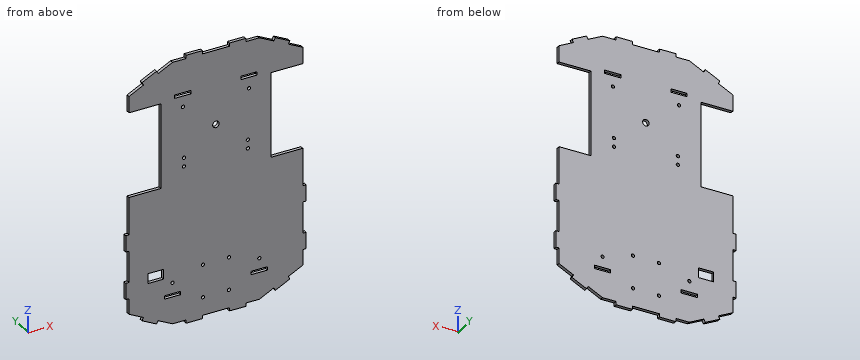
from build123d import *

# Parameters (mm, degrees)
SKETCH1_R           = 1.5
SKETCH1_R_2         = 3
SKETCH1_W           = 15.1
SKETCH1_H           = 3.1
SKETCH1_W_2         = 14
SKETCH1_H_2         = 9
BOSS_EXTRUDE1_DEPTH = 3


with BuildPart() as part:
    # Sketch1 → Boss-Extrude1 (new body)
    with BuildSketch(Plane(origin=(0, 0, 0), x_dir=(1, 0, 0), z_dir=(0, 1, 0))):
        Polygon((120, 0), (133.291796068, 6.645898034), (134.633436854, 3.962616461), (148.049844719, 10.670820393), (146.708203932, 13.354101966), (160, 20), (160, 35), (130.7, 35), (130.7, 112.71), (160, 112.71), (160, 147.0325), (163, 147.0325), (163, 162.0325), (160, 162.0325), (160, 190.6775), (163, 190.6775), (163, 205.6775), (160, 205.6775), (160, 220), (146.708203932, 226.645898034), (148.049844719, 229.329179607), (134.633436854, 236.037383539), (133.291796068, 233.354101966), (120, 240), (107.5, 240), (107.5, 243), (92.5, 243), (92.5, 240), (67.5, 240), (67.5, 243), (52.5, 243), (52.5, 240), (40, 240), (26.708203932, 233.354101966), (25.366563146, 236.037383539), (11.950155281, 229.329179607), (13.291796068, 226.645898034), (0, 220), (0, 205.6775), (-3, 205.6775), (-3, 190.6775), (0, 190.6775), (0, 162.0325), (-3, 162.0325), (-3, 147.0325), (0, 147.0325), (0, 112.71), (29.3, 112.71), (29.3, 35), (0, 35), (0, 20), (13.291796068, 13.354101966), (11.950155281, 10.670820393), (25.366563146, 3.962616461), (26.708203932, 6.645898034), (40, 0), (52.5, 0), (52.5, -3), (67.5, -3), (67.5, 0), (92.5, 0), (92.5, -3), (107.5, -3), (107.5, 0), align=None)
        with Locations(Location((50.6, 98.52, 0), (0, 0, 270))):
            Circle(SKETCH1_R, mode=Mode.SUBTRACT)
        with Locations(Location((50.6, 90.52, 0), (0, 0, 270))):
            Circle(SKETCH1_R, mode=Mode.SUBTRACT)
        with Locations(Location((68.025, 223.5, 0), (0, 0, 270))):
            Circle(SKETCH1_R, mode=Mode.SUBTRACT)
        with Locations(Location((68.025, 193.55, 0), (0, 0, 270))):
            Circle(SKETCH1_R, mode=Mode.SUBTRACT)
        with Locations(Location((91.975, 193.55, 0), (0, 0, 90))):
            Circle(SKETCH1_R, mode=Mode.SUBTRACT)
        with Locations(Location((91.975, 223.5, 0), (0, 0, 90))):
            Circle(SKETCH1_R, mode=Mode.SUBTRACT)
        with Locations(Location((109.4, 90.52, 0), (0, 0, 90))):
            Circle(SKETCH1_R, mode=Mode.SUBTRACT)
        with Locations(Location((109.4, 98.52, 0), (0, 0, 90))):
            Circle(SKETCH1_R, mode=Mode.SUBTRACT)
        with Locations(Location((40.05, 202.335880608, 0), (0, 0, 270))):
            Circle(SKETCH1_R, mode=Mode.SUBTRACT)
        with Locations(Location((49.592731594, 43.515235673, 0), (0, 0, 270))):
            Circle(SKETCH1_R, mode=Mode.SUBTRACT)
        with Locations(Location((110.407268406, 43.515235673, 0), (0, 0, 90))):
            Circle(SKETCH1_R, mode=Mode.SUBTRACT)
        with Locations(Location((119.95, 202.335880608, 0), (0, 0, 90))):
            Circle(SKETCH1_R, mode=Mode.SUBTRACT)
        with Locations(Location((80, 68.197866296, 0), (0, 0, 270))):
            Circle(SKETCH1_R_2, mode=Mode.SUBTRACT)
        with Locations((40, 213.785880608)):
            Rectangle(SKETCH1_W, SKETCH1_H, mode=Mode.SUBTRACT)
        with Locations((49.542731594, 32.073098627)):
            Rectangle(SKETCH1_W, SKETCH1_H, mode=Mode.SUBTRACT)
        with Locations((120, 213.785880608)):
            Rectangle(SKETCH1_W, SKETCH1_H, mode=Mode.SUBTRACT)
        with Locations((110.457268406, 32.073098627)):
            Rectangle(SKETCH1_W, SKETCH1_H, mode=Mode.SUBTRACT)
        with Locations((24.658359214, 192.159143415)):
            Rectangle(SKETCH1_W_2, SKETCH1_H_2, mode=Mode.SUBTRACT)
    extrude(amount=BOSS_EXTRUDE1_DEPTH)


solid = part.part
For this review, take the finished solid that the model builds, in its own axes (mm). Coordinates: 2 decimals unless noted, no trailing zeros. Loops run counter-clockwise (first coordinate to the right, second up) from the corner with the lowest first, then second, coordinate; pieces in that order, holes last. Notation, with made-up numbers: (43, -31) - (84, -31) arc R21 cw to (84, -20) - close; hole circle Ø9 at (85, 71.25). An arc over 180 degrees is marked (long way). Use a Markdown table: item, result. Add a question column.
Item 1: We need section A-A (z = -86). Give the boundary of the cut face in (x, y).
Item 2: Insertion check: pin 1 Ø1.5 at (x, y) = (116, 1.5) entering from -Z; pin 2 Ø0.9 at (x, y) = (46, 2) entering from +Z; pin 3 Ø0.9 at (x, y) = (-1.5, 1) entering from -Z. Each pin has a flat end and moves straight along its axis. Give the tip position at first contact, or say it passes through.
Item 3: For line 1 (X direction, y = 2.3, z = -98.52); line 2 (X direction, y = 0.6, z = -193.55) (3 decimals); line 3 (Z direction, x = 45, y = 1.55), list the stretches that pass through material, from the lowest coordinate up.
Item 4: We need section B-B (y = 1.35). Give the number of separate pieces and of enclosed holes in the cut face, and give its area (3 significant figures).
Results list:
| question | item | result |
|---|---|---|
| 1 | outline | (29.3, 0) - (130.7, 0) - (130.7, 3) - (29.3, 3) - close |
| 2 | pin 1 | stops at z = -240 |
| 2 | pin 2 | stops at z = 0 |
| 2 | pin 3 | stops at z = -205.68 |
| 3 | line 1 | x = 29.3 to 49.1, 52.1 to 107.9, 110.9 to 130.7 |
| 3 | line 2 | x = -3 to 17.658, 31.658 to 66.525, 69.525 to 90.475, 93.475 to 163 |
| 3 | line 3 | z = -240 to -215.34, -212.24 to -33.62, -30.52 to 0 |
| 4 | separate pieces | 1 |
| 4 | enclosed holes | 18 |
| 4 | area | 32,400 mm^2 |
